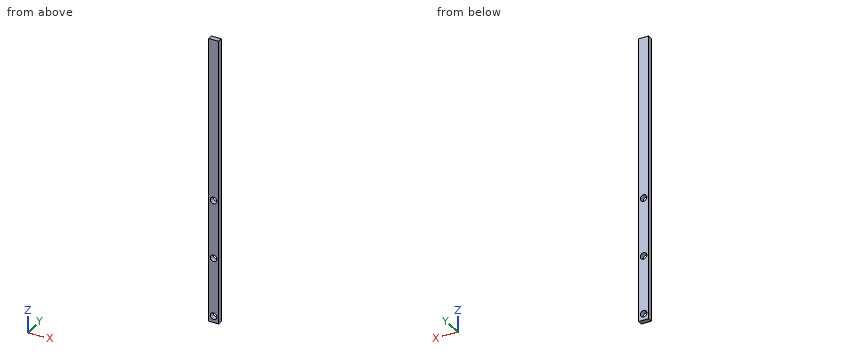
```python
from build123d import *

# Parameters (mm, degrees)
F0_W     = 38.1
F0_H     = 500
F1_DEPTH = 19.05
F2_R     = 12.7
F3_DEPTH = 25
F4_R     = 12.7
F5_DEPTH = 25
F6_W     = 38.1
F6_H     = 19.05
F7_DEPTH = 600


with BuildPart() as f1:
    # F0 (on Front) → F1 (new body)
    with BuildSketch(Plane.XZ):
        with Locations((19.05, 250)):
            Rectangle(F0_W, F0_H)
    extrude(amount=F1_DEPTH)

    # F2 (on face) → F3 (cut)
    with BuildSketch(Plane.XZ.offset(19.05)):
        with Locations((19.05, 475)):
            Circle(F2_R)
        with Locations((19.05, 25)):
            Circle(F2_R)
    extrude(amount=-F3_DEPTH, mode=Mode.SUBTRACT)

    # F4 (on face) → F5 (cut)
    with BuildSketch(Plane.XZ.offset(19.05)):
        with Locations((19.05, 250)):
            Circle(F4_R)
    extrude(amount=-F5_DEPTH, mode=Mode.SUBTRACT)

    # F6 (on face) → F7 (join)
    with BuildSketch(Plane.XY.offset(500)):
        with Locations((19.05, -9.525)):
            Rectangle(F6_W, F6_H)
    extrude(amount=F7_DEPTH)


solid = f1.part
```
The model under review builds one solid part; all positions refer to its coordinate system, in mm. Coordinates: 2 decimals unless noted, no trailing zeros. Order: outer loops, then holes, each group sorted by start corner. A loop starts at its lowest first (then second) coordinate and runs counter-clockwise, first axis right, second up. Notation, with made-up numbers: M 53,-13.75 L 67,-13.75 A27 cw 67,6.25 Z; hole C -4,-6 d6. An arc over 180 degrees is marked long. One line per question, with ' | ' between items.
(1) For probe 1 along Z at (x, y) = (19.05, -7.75); probe 2 along Z at (x, y) = (17, -1.25), list the stretches that pass through material, from the lowest coordinate up. Write a range as from..to.
Geometry results:
probe 1: z = 0..12.3, 37.7..237.3, 262.7..462.3, 487.7..1100 | probe 2: z = 0..12.47, 37.53..237.47, 262.53..462.47, 487.53..1100
(2) Add section C-C, the plane y = -4.25. Write out the cut boundary in (x, z).
Geometry results:
outline: M 0,0 L 38.1,0 L 38.1,1100 L 0,1100 Z; hole C 19.05,25 d25.4; hole C 19.05,250 d25.4; hole C 19.05,475 d25.4
(3) Add section B-B, the plane z = 25. Write out the cut boundary in (x, y), then the cut area to 3 significant figures.
Geometry results:
outline: M 0,-19.05 L 6.35,-19.05 L 6.35,0 L 0,0 Z; M 31.75,-19.05 L 38.1,-19.05 L 38.1,0 L 31.75,0 Z | area: 242 mm²
(4) Add section A-A, the plane x = 19.05. Write out the cut boundary in (y, z).
Geometry results:
outline: M -19.05,0 L 0,0 L 0,12.3 L -19.05,12.3 Z; M -19.05,37.7 L 0,37.7 L 0,237.3 L -19.05,237.3 Z; M -19.05,262.7 L 0,262.7 L 0,462.3 L -19.05,462.3 Z; M -19.05,487.7 L 0,487.7 L 0,1100 L -19.05,1100 Z
